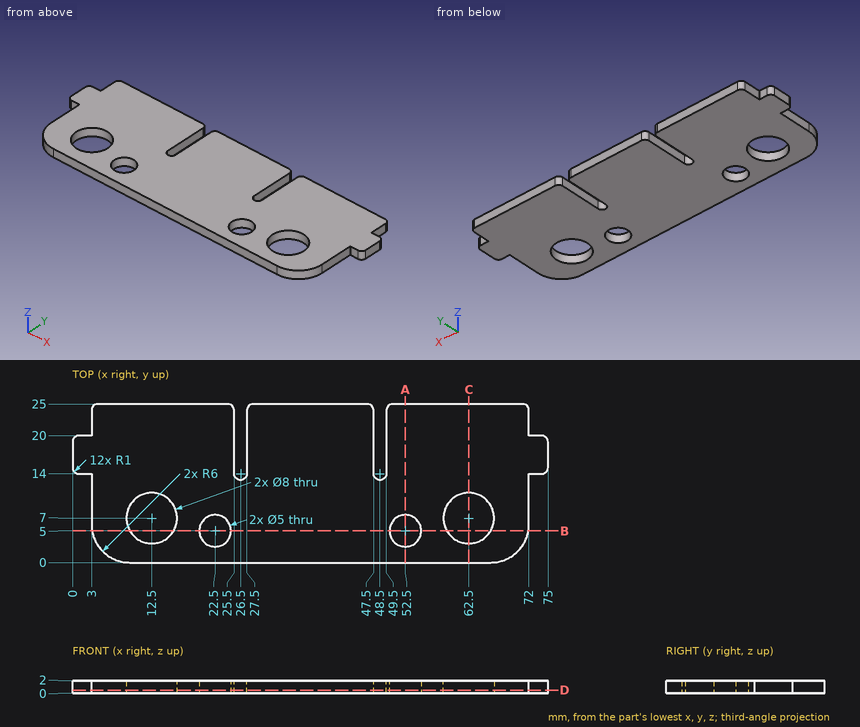
Geometry check sheet. Reference: drawing and pictorial views, mm from the part's lowest x, y, z. Give positions to 0.01 mm unless a question says otherwise; leave off trailing zeros. Write each loop counter-clockwise with the first axis right and the second up, starting at its lowest first coordinate (ties: lowest second). Pieces come first, ordered by that corner, then holes. Notation, with made-up numbers: (44, -16.75) -> (57, -16.75) arc R15 ccw to (57, 9.25) -> close; hole circle Ø1 at (71.25, 13). An arc over 180 degrees is marked (long way). One line per item, written item: value. Start each with the question number.
Item 1: Section check C-C on x = 62.5. Record the cut outline in (y, z), then the cut area to 3 significant figures.
Item 2: Gauge pin test, flat ends, axial feed: pin 1 (1 mm diameter, centred on y = 9.5, z = 1, fed in from +X); pin 2 (1 mm diameter, centred on y = 21, z = 0.5, fed in from -X); pin 3 (0.6 mm diameter, centred on x = 72.5, z = 1, fed in from -Y). Record the tip position at first contact, or that the pin passes through.
Item 3: Section check A-A on x = 52.5. Record the cut outline in (y, z).
Item 4: Material ranges on probe 1 along X at (y, z) = (16.75, 1.5); probe 2 along X at (y, z) = (20.75, 1.45); probe 3 along Y at (x, z) = (52.5, 0.6), recorded low to high. Write a range as from..to.
Item 5: Section check B-B on y = 5. Record the cut outline in (x, z).
Item 6: Section check D-D on z = 0.5. State how many separate pieces and enclosed holes the cut face has, then the cut area to 3 significant figures.
Results list:
1. outline: (0, 0) -> (3, 0) -> (3, 2) -> (0, 2) -> close; (11, 0) -> (25, 0) -> (25, 2) -> (11, 2) -> close
1. area: 34.0 mm²
2. pin 1: x = 72
2. pin 2: x = 3
2. pin 3: y = 14
3. outline: (0, 0) -> (2.5, 0) -> (2.5, 2) -> (0, 2) -> close; (7.5, 0) -> (25, 0) -> (25, 2) -> (7.5, 2) -> close
4. probe 1: 0..25.5, 27.5..47.5, 49.5..75
4. probe 2: 3..25.5, 27.5..47.5, 49.5..72
4. probe 3: 0..2.5, 7.5..25
5. outline: (3.08, 0) -> (9.04, 0) -> (9.04, 2) -> (3.08, 2) -> close; (15.96, 0) -> (20, 0) -> (20, 2) -> (15.96, 2) -> close; (25, 0) -> (50, 0) -> (50, 2) -> (25, 2) -> close; (55, 0) -> (59.04, 0) -> (59.04, 2) -> (55, 2) -> close; (65.96, 0) -> (71.92, 0) -> (71.92, 2) -> (65.96, 2) -> close
6. separate pieces: 1
6. enclosed holes: 4
6. area: 1,560 mm²
